Read the model definition and answer for the solid it produces. Units are mm, in the model's axes. A direction names the side the tool comes from. Round coordinates to 2 decimals unless told otherwise and drop trailing zeros.
from build123d import *

# Parameters (mm, degrees)
IZIM1_W                      = 78
IZIM1_H                      = 78
Y_KSEKLIK_EKSTR_ZYON1_DEPTH  = 3
Y_KSEKLIK_EKSTR_ZYON5_DEPTH  = 19.5
IZIM10_R                     = 2
KES_EKSTR_ZYON3_DEPTH        = 26.5
IZIM18_W                     = 78
IZIM18_H                     = 78
Y_KSEKLIK_EKSTR_ZYON8_DEPTH  = 3
DIK_W                        = 15
DIK_H                        = 4
Y_KSEKLIK_EKSTR_ZYON12_DEPTH = 22
YANDESTEK_W                  = 4
YANDESTEK_H                  = 13.5
Y_KSEKLIK_EKSTR_ZYON13_DEPTH = 10
IZIM23_R                     = 2.05
KES_EKSTR_ZYON4_DEPTH        = 14
IZIM24_R                     = 2.05
KES_EKSTR_ZYON5_DEPTH        = 14
IZIM25_R                     = 2.05
KES_EKSTR_ZYON6_DEPTH        = 14
IZIM26_R                     = 2.05
KES_EKSTR_ZYON7_DEPTH        = 14
IZIM27_R                     = 2.05
KES_EKSTR_ZYON8_DEPTH        = 14
IZIM28_W                     = 78
IZIM28_H                     = 94
Y_KSEKLIK_EKSTR_ZYON15_DEPTH = 3
IZIM29_R                     = 2
KES_EKSTR_ZYON9_DEPTH        = 3
IZIM30_R                     = 2
Y_KSEKLIK_EKSTR_ZYON16_DEPTH = 19
IZIM31_R                     = 7.5
KES_EKSTR_ZYON10_DEPTH       = 19
KES_EKSTR_ZYON11_START       = -19
IZIM32_R                     = 2
KES_EKSTR_ZYON11_DEPTH       = 19
RADYUS1_R                    = 25
RADYUS2_R                    = 20


with BuildPart() as part:
    # Çizim1 → Yükseklik-Ekstrüzyon1 (new body)
    with BuildSketch(Plane(origin=(0, 0, 0), x_dir=(1, 0, 0), z_dir=(0, 1, 0))):
        with Locations((0, -9)):
            Rectangle(IZIM1_W, IZIM1_H)
    extrude(amount=Y_KSEKLIK_EKSTR_ZYON1_DEPTH)

    # Çizim9 → Yükseklik-Ekstrüzyon5 (add)
    with BuildSketch(Plane(origin=(0, 3, 0), x_dir=(1, 0, 0), z_dir=(0, 1, 0))):
        with BuildLine():
            Line((-14.722431864, -17.5), (-11.747340124, -17.5))
            ThreePointArc((-11.747340124, -17.5), (0, 5.5), (11.747340124, -17.5))
            Line((11.747340124, -17.5), (14.722431864, -17.5))
            ThreePointArc((14.722431864, -17.5), (15.595161026, -15.766901254), (16.264705882, -13.945638741))
            ThreePointArc((16.264705882, -13.945638741), (22, -9), (16.264705882, -4.054361259))
            ThreePointArc((16.264705882, -4.054361259), (0, 8), (-16.264705882, -4.054361259))
            ThreePointArc((-16.264705882, -4.054361259), (-22, -9), (-16.264705882, -13.945638741))
            ThreePointArc((-16.264705882, -13.945638741), (-15.595161026, -15.766901254), (-14.722431864, -17.5))
        make_face()
    extrude(amount=Y_KSEKLIK_EKSTR_ZYON5_DEPTH)

    # Çizim10 → Kes-Ekstrüzyon3 (cut)
    with BuildSketch(Plane(origin=(0, 22.5, 0), x_dir=(1, 0, 0), z_dir=(0, 1, 0))):
        with Locations(Location((-18.25, -9, 0), (0, 0, 270))):
            Circle(IZIM10_R)
        with Locations(Location((18.25, -9, 0), (0, 0, 270))):
            Circle(IZIM10_R)
    extrude(amount=-KES_EKSTR_ZYON3_DEPTH, mode=Mode.SUBTRACT)

    # Çizim18 → Yükseklik-Ekstrüzyon8 (add)
    with BuildSketch(Plane(origin=(0, 0, 0), x_dir=(1, 0, 0), z_dir=(0, 1, 0))):
        with Locations((0, 69)):
            Rectangle(IZIM18_W, IZIM18_H)
    extrude(amount=Y_KSEKLIK_EKSTR_ZYON8_DEPTH)

    # dik → Yükseklik-Ekstrüzyon12 (add)
    with BuildSketch(Plane(origin=(0, 3, 0), x_dir=(1, 0, 0), z_dir=(0, 1, 0))):
        with Locations((0, 34.5)):
            Rectangle(DIK_W, DIK_H)
        with Locations((0, 25)):
            Rectangle(DIK_W, DIK_H)
        Polygon((33.346991903, 17.721061161), (37.982246819, 3.455213417), (34.178020754, 2.219145439), (29.542765838, 16.484993184), align=None)
        Polygon((24.311954998, 14.785399715), (20.507728933, 13.549331737), (25.142983849, -0.716516007), (28.947209914, 0.51955197), align=None)
        Polygon((28.109574419, -26.929747897), (15.974319503, -35.746526681), (13.623178494, -32.510458704), (25.75843341, -23.693679919), align=None)
        Polygon((22.525614522, -19.24408645), (20.174473513, -16.008018473), (10.390359606, -23.116593325), (10.390359606, -28.060865235), align=None)
        Polygon((-15.974319503, -35.746526681), (-28.109574419, -26.929747897), (-25.75843341, -23.693679919), (-13.623178494, -32.510458704), align=None)
        Polygon((-10.390359606, -23.116593325), (-20.174473513, -16.008018473), (-22.525614522, -19.24408645), (-10.390359606, -28.060865235), align=None)
        Polygon((-37.982246819, 3.455213417), (-33.346991903, 17.721061161), (-29.542765838, 16.484993184), (-34.178020754, 2.219145439), align=None)
        Polygon((-28.947209914, 0.51955197), (-25.142983849, -0.716516007), (-20.507728933, 13.549331737), (-24.311954998, 14.785399715), align=None)
    extrude(amount=Y_KSEKLIK_EKSTR_ZYON12_DEPTH)

    # yandestek → Yükseklik-Ekstrüzyon13 (add)
    with BuildSketch(Plane(origin=(0, 3, 0), x_dir=(1, 0, 0), z_dir=(0, 1, 0))):
        Polygon((-37.982246819, 3.455213417), (-25.142983849, -0.716516007), (-26.379051826, -4.520742072), (-37.982246819, -0.75063548), align=None)
        Polygon((-20.174473513, -16.008018473), (-28.109574419, -26.929747897), (-31.345642396, -24.578606888), (-23.41054149, -13.656877464), align=None)
        Polygon((-20.507728933, 13.549331737), (-33.346991903, 17.721061161), (-32.110923926, 21.525287226), (-19.271660956, 17.353557802), align=None)
        with Locations((-9.5, 29.75)):
            Rectangle(YANDESTEK_W, YANDESTEK_H)
        with Locations((9.5, 29.75)):
            Rectangle(YANDESTEK_W, YANDESTEK_H)
        Polygon((32.110923926, 21.525287226), (33.346991903, 17.721061161), (20.507728933, 13.549331737), (19.271660956, 17.353557802), align=None)
        Polygon((37.982246819, 3.455213417), (37.982246819, -0.75063548), (26.379051826, -4.520742072), (25.142983849, -0.716516007), align=None)
        Polygon((31.345642396, -24.578606888), (28.109574419, -26.929747897), (20.174473513, -16.008018473), (23.41054149, -13.656877464), align=None)
    extrude(amount=Y_KSEKLIK_EKSTR_ZYON13_DEPTH)

    # Çizim23 → Kes-Ekstrüzyon4 (cut)
    with BuildSketch(Plane(origin=(-22.517475219, 0, 30.992645786), x_dir=(0.8090169943749423, 0, 0.5877852522924801), z_dir=(-0.5877852522924801, 0, 0.8090169943749423))):
        with Locations((0.587785252, 20.9)):
            Circle(IZIM23_R)
    extrude(amount=-KES_EKSTR_ZYON4_DEPTH, mode=Mode.SUBTRACT)

    # Çizim24 → Kes-Ekstrüzyon5 (cut)
    with BuildSketch(Plane(origin=(22.517475219, 0, 30.992645786), x_dir=(0.8090169943749507, 0, -0.5877852522924687), z_dir=(0.5877852522924687, 0, 0.8090169943749507))):
        with Locations((-0.587785252, 20.9)):
            Circle(IZIM24_R)
    extrude(amount=-KES_EKSTR_ZYON5_DEPTH, mode=Mode.SUBTRACT)

    # Çizim25 → Kes-Ekstrüzyon6 (cut)
    with BuildSketch(Plane(origin=(35.370726735, 0, -11.492645786), x_dir=(-0.30901699437494434, 0, -0.9510565162951546), z_dir=(0.9510565162951545, 0, -0.3090169943749443))):
        with Locations((-0.951056516, 20.9)):
            Circle(IZIM25_R)
    extrude(amount=-KES_EKSTR_ZYON6_DEPTH, mode=Mode.SUBTRACT)

    # Çizim26 → Kes-Ekstrüzyon7 (cut)
    with BuildSketch(Plane(origin=(0, 0, -36.5), x_dir=(-1, 0, 0), z_dir=(0, 0, -1))):
        with Locations((0, 20.9)):
            Circle(IZIM26_R)
    extrude(amount=-KES_EKSTR_ZYON7_DEPTH, mode=Mode.SUBTRACT)

    # Çizim27 → Kes-Ekstrüzyon8 (cut)
    with BuildSketch(Plane(origin=(-35.370726735, 0, -11.492645786), x_dir=(-0.30901699437494806, 0, 0.9510565162951534), z_dir=(-0.9510565162951534, 0, -0.30901699437494806))):
        with Locations((0.951056516, 20.9)):
            Circle(IZIM27_R)
    extrude(amount=-KES_EKSTR_ZYON8_DEPTH, mode=Mode.SUBTRACT)

    # Çizim28 → Yükseklik-Ekstrüzyon15 (add)
    with BuildSketch(Plane(origin=(0, 3, 0), x_dir=(1, 0, 0), z_dir=(0, 1, 0))):
        with Locations((0, 155)):
            Rectangle(IZIM28_W, IZIM28_H)
    extrude(amount=-Y_KSEKLIK_EKSTR_ZYON15_DEPTH)

    # Çizim29 → Kes-Ekstrüzyon9 (cut)
    with BuildSketch(Plane(origin=(0, 3, 0), x_dir=(1, 0, 0), z_dir=(0, 1, 0))):
        with Locations(Location((-9.5, 161.5, 0), (0, 0, 270))):
            Circle(IZIM29_R)
        with Locations(Location((9.5, 161.5, 0), (0, 0, 270))):
            Circle(IZIM29_R)
        with Locations(Location((-24.5, 176.5, 0), (0, 0, 270))):
            Circle(IZIM29_R)
        with Locations(Location((24.5, 176.5, 0), (0, 0, 270))):
            Circle(IZIM29_R)
    extrude(amount=-KES_EKSTR_ZYON9_DEPTH, mode=Mode.SUBTRACT)

    # Çizim30 → Yükseklik-Ekstrüzyon16 (add)
    with BuildSketch(Plane(origin=(0, 3, 0), x_dir=(1, 0, 0), z_dir=(0, 1, 0))):
        with BuildLine():
            Line((-15.782902141, 202), (-12.986435231, 202))
            ThreePointArc((-12.986435231, 202), (0, 181.05), (12.986435231, 202))
            Line((12.986435231, 202), (15.782902141, 202))
            ThreePointArc((15.782902141, 202), (16.314196986, 200.504742849), (16.704178082, 198.966567663))
            ThreePointArc((16.704178082, 198.966567663), (22, 195.55), (16.704178082, 192.133432337))
            ThreePointArc((16.704178082, 192.133432337), (0, 178.5), (-16.704178082, 192.133432337))
            ThreePointArc((-16.704178082, 192.133432337), (-22, 195.55), (-16.704178082, 198.966567663))
            ThreePointArc((-16.704178082, 198.966567663), (-16.314196986, 200.504742849), (-15.782902141, 202))
        make_face()
        with Locations(Location((-18.25, 195.55, 0), (0, 0, 270))):
            Circle(IZIM30_R, mode=Mode.SUBTRACT)
        with Locations(Location((18.25, 195.55, 0), (0, 0, 270))):
            Circle(IZIM30_R, mode=Mode.SUBTRACT)
    extrude(amount=Y_KSEKLIK_EKSTR_ZYON16_DEPTH)

    # Çizim31 → Kes-Ekstrüzyon10 (cut)
    with BuildSketch(Plane(origin=(0, 3, 0), x_dir=(1, 0, 0), z_dir=(0, 1, 0))):
        with Locations(Location((0, -9, 0), (0, 0, 270))):
            Circle(IZIM31_R)
        with Locations((0, 195.55)):
            Circle(IZIM31_R)
    extrude(amount=-KES_EKSTR_ZYON10_DEPTH, mode=Mode.SUBTRACT)

    # Çizim32 → Kes-Ekstrüzyon11 (cut)
    with BuildSketch(Plane(origin=(0, 3, 0), x_dir=(1, 0, 0), z_dir=(0, 1, 0)).offset(KES_EKSTR_ZYON11_START)):
        with Locations(Location((-29, 182, 0), (0, 0, 270))):
            Circle(IZIM32_R)
        with Locations(Location((29, 182, 0), (0, 0, 270))):
            Circle(IZIM32_R)
        with Locations(Location((-18.25, 195.55, 0), (0, 0, 90))):
            Circle(IZIM32_R)
        with Locations(Location((18.25, 195.55, 0), (0, 0, 90))):
            Circle(IZIM32_R)
        with Locations(Location((-29, -38, 0), (0, 0, 270))):
            Circle(IZIM32_R)
        with Locations(Location((29, -38, 0), (0, 0, 270))):
            Circle(IZIM32_R)
        with Locations(Location((-29, 72, 0), (0, 0, 270))):
            Circle(IZIM32_R)
        with Locations(Location((29, 72, 0), (0, 0, 270))):
            Circle(IZIM32_R)
    extrude(amount=KES_EKSTR_ZYON11_DEPTH, mode=Mode.SUBTRACT)

    # Radyus1
    radyus1_edges = [part.edges().sort_by_distance(p)[0] for p in [
        (-39, 1.5, -202),
        (39, 1.5, -202),
    ]]
    fillet(radyus1_edges, radius=RADYUS1_R)

    # Radyus2
    radyus2_edges = [part.edges().sort_by_distance(p)[0] for p in [
        (39, 1.5, 48),
        (-39, 1.5, 48),
    ]]
    fillet(radyus2_edges, radius=RADYUS2_R)


solid = part.part
Q1. Section A-A (y = 15.5) is taken. State how many separate pieces and enclosed holes the cut face has, then the cut area to 3 significant figures.
Verdict:
separate pieces: 12
enclosed holes: 4
area: 1,010 mm2
Q2. Straight lines are drawn through the part: probe 1 along X at (y, z) = (16.5, 9); probe 2 along Z at (x, y) = (-29, 1); probe 3 along X at (y, z) = (17, 7.5). For each, find the intervals that lie inside material, in ascending order.
Verdict:
probe 1: x = -22 to -20.25, -16.25 to -14.5, 14.5 to 16.25, 20.25 to 22
probe 2: z = -197 to -184, -180 to -74, -70 to 36, 40 to 45.32
probe 3: x = -21.77 to -19.57, -16.93 to -14.42, 14.42 to 16.93, 19.57 to 21.77
Q3. Determine the mould class of faces 5 (the cylindrical face through (-22.105, 22.285, 28.855)), 6 (the flat face through (-26.891, 7.93, -15.623)), 7 (the flat face through (32, 13, 0)) for opening direction Y: pulls with the +Y half, pulls with the -Y half, needs draft (parallel to the pull), parting line crosses it, or undercut.
Verdict:
face 5: undercut
face 6: needs draft
face 7: pulls with the +Y half
Q4. Which of the six approach directions +Z, -Z, +X, -X, +Y, -Y give full straight-line access (tool end or side, diameter ignored) to faces 1 (the flat face through (7.5, 19, -34)), 2 (the flat face through (-10.39, 14, 26)), 3 (the flat face through (31.893, 13.846, -9.252)), 4 (the flat face through (-10, 13, -30))?
Verdict:
face 1: +X, +Y
face 2: +Z, +Y
face 3: +Y
face 4: -X, +Y
Q5. Flat-ended cylindrical pins translate along their axes: pin 1 Ø4 at (x, y) = (-30, 5.5) entering from -Z; pin 2 Ø6 at (x, y) = (28, 12.5) entering from -Z; pin 3 Ø12 at (x, y) = (0, 11.5) entering from -Z. Find the tip coordinate at first contact, or state that the pin passes through.
Verdict:
pin 1: stops at z = -21.49
pin 2: stops at z = -21.16
pin 3: stops at z = -182.35
